The model under review builds one solid part; all positions refer to its coordinate system, in mm. A direction names the side the tool comes from. Round coordinates to 2 decimals unless told otherwise and drop trailing zeros. Write each loop counter-clockwise with the first axis right and the second up, starting at its lowest first coordinate (ties: lowest second). Pieces come first, ordered by that corner, then holes.
Item 1: Clearance check with flat-ended pins moving along their axes: pin 1 Ø2 at (x, z) = (3, -18) entering from +Y; pin 2 Ø10 at (x, z) = (1.5, -8) entering from -Y; pin 3 Ø1.6 at (x, z) = (0, -14.75) entering from +Y. State where each tip first meets the part, or that it passes through.
Item 2: To check wall thickness, follow L1, parallel to Y at x = 5.6, z = -5; L2, parallel to X at y = -5.6, z = -5; L3, parallel to X at y = 12.5, z = -3. State the ranges of each line that lie inside material, in increasing order.
Item 3: Draft analysis for pull direction Z (two halves, no side actions). For faces 1 (the face through (-0.492, -3.948, -15.521)), 2 (the face through (5, 0, -20)), 3 (the face through (3.948, 8.939, -5.422)), state which applies: +Z half, -Z half, draft (parallel to the pull), parting line (faces both ways), or undercut.
Item 4: Machinability: for faces 4 (the face through (0, 10, 0.5)), 5 (the face through (5, 2.75, -15)), 6 (the face through (4.4, -2.81, -10.22)), 7 (the face through (3.5, 0, -15)), which of the approach directions +Z, -Z, +X, -X, +Y, -Y give a long, thin tool a straight path to every point of the face, cutting with its end or side? Answer none if there is none.
Item 5: Add section A-A (y = 11.75). Give the boundary of the cut face in (x, z).
```python
from build123d import *

# Parameters (mm, degrees)
BOSS_EXTRUDE1_DEPTH           = 0.5
SKETCH6_R                     = 1.1
BOSS_EXTRUDE3_DEPTH           = 1.5
BOSS_EXTRUDE3_TAPER           = 10
BOSS_EXTRUDE3_OTHER_WAY_DEPTH = 1.5
BOSS_EXTRUDE3_OTHER_WAY_TAPER = 10
CHAMFER1_SIZE                 = 0.24656061
CHAMFER1_SIZE_2               = 0.2
CIRPATTERN2_COUNT             = 2
CIRPATTERN2_ANGLE             = 270
CIRPATTERN3_COUNT             = 2
CIRPATTERN3_ANGLE             = 90
CUT_EXTRUDE8_DEPTH            = 33.330326321
CUT_EXTRUDE10_DEPTH           = 30.5
CUT_EXTRUDE11_DEPTH           = 33.330326321
SKETCH8_R                     = 1.35
SKETCH8_R_2                   = 1.01183651
BOSS_EXTRUDE4_DEPTH           = 0.15
SKETCH12_R                    = 1.35
SKETCH12_R_2                  = 1.01183651
BOSS_EXTRUDE5_DEPTH           = 0.15
SKETCH13_R                    = 1.35
SKETCH13_R_2                  = 1.01183651
BOSS_EXTRUDE6_DEPTH           = 0.15
SKETCH2_R                     = 1.35
BOSS_EXTRUDE2_DEPTH           = 1
FILLET1_R                     = 1
CUT_EXTRUDE2_DEPTH            = 34.638240887
CUT_EXTRUDE4_DEPTH            = 32.129266776
CUT_EXTRUDE6_DEPTH            = 4


with BuildPart() as part:
    # Sketch1 → Boss-Extrude1 (new, symmetric)
    with BuildSketch(Plane.XY):
        Polygon((-5, 2.75), (-5, 5), (-2.75, 5), (-2.75, 15), (2.75, 15), (2.75, 5), (-5, -2.75), (-15, -2.75), (-15, 2.75), align=None)
    extrude(amount=BOSS_EXTRUDE1_DEPTH, both=True)

    # Sketch6 → Boss-Extrude3 (add)
    with BuildSketch(Plane(origin=(0, -0.5, 0), x_dir=(-1, 0, 0), z_dir=(0, 0, -1))):
        with Locations((0, 10.25)):
            Circle(SKETCH6_R)
        with Locations((9.75, 0.5)):
            Circle(SKETCH6_R)
    extrude(amount=BOSS_EXTRUDE3_DEPTH, taper=BOSS_EXTRUDE3_TAPER)

    # Sketch6 → Boss-Extrude3 other way (add)
    with BuildSketch(Plane(origin=(0, -0.5, 0), x_dir=(-1, 0, 0), z_dir=(0, 0, -1))):
        with Locations((0, 10.25)):
            Circle(SKETCH6_R)
        with Locations((9.75, 0.5)):
            Circle(SKETCH6_R)
    extrude(amount=-BOSS_EXTRUDE3_OTHER_WAY_DEPTH, taper=BOSS_EXTRUDE3_OTHER_WAY_TAPER)

    # Chamfer1
    # the kernel refuses this chamfer: 0.24656061, 0.2 mm, written as the material it takes off along each edge
    with BuildSketch(Plane(origin=(0, 9.75, 1.5), x_dir=(-1, 0, 0), z_dir=(0, -1, 0))) as chamfer1_piece_1:
        Polygon((0.835509529 + CHAMFER1_SIZE * 0.173648177924, CHAMFER1_SIZE * 0.984807754467), (0.835509529 - CHAMFER1_SIZE_2, 0), (0.835509529, 0), align=None)
    revolve(axis=Axis((0, 9.75, 1.5), (0, 0, -1)), mode=Mode.SUBTRACT)
    with BuildSketch(Plane(origin=(0, 9.75, -1.5), x_dir=(-1, 0, 0), z_dir=(0, 1, 0))) as chamfer1_piece_2:
        Polygon((0.835509529 + CHAMFER1_SIZE_2 * 0.173648177667, CHAMFER1_SIZE_2 * 0.984807753012), (0.835509529 - CHAMFER1_SIZE * 1.00000000148, 0), (0.835509529, 0), align=None)
    revolve(axis=Axis((0, 9.75, -1.5), (0, 0, 1)), mode=Mode.SUBTRACT)
    with BuildSketch(Plane(origin=(-9.75, 0, 1.5), x_dir=(-1, 0, 0), z_dir=(0, -1, 0))) as chamfer1_piece_3:
        Polygon((0.835509529 + CHAMFER1_SIZE * 0.173648177924, CHAMFER1_SIZE * 0.984807754467), (0.835509529 - CHAMFER1_SIZE_2, 0), (0.835509529, 0), align=None)
    revolve(axis=Axis((-9.75, 0, 1.5), (0, 0, -1)), mode=Mode.SUBTRACT)
    with BuildSketch(Plane(origin=(-9.75, 0, -1.5), x_dir=(-1, 0, 0), z_dir=(0, 1, 0))) as chamfer1_piece_4:
        Polygon((0.835509529 + CHAMFER1_SIZE_2 * 0.173648177667, CHAMFER1_SIZE_2 * 0.984807753012), (0.835509529 - CHAMFER1_SIZE * 1.00000000148, 0), (0.835509529, 0), align=None)
    revolve(axis=Axis((-9.75, 0, -1.5), (0, 0, 1)), mode=Mode.SUBTRACT)


with BuildPart() as cirpattern2_1:
    # CirPattern2: pattern copy
    add(part.part.rotate(Axis((0, -5, 0), (1, 0, 0)), 1 * CIRPATTERN2_ANGLE / (CIRPATTERN2_COUNT - 1)))

    # Sketch9 → Cut-Extrude8 (cut, through all)
    with BuildSketch(Plane.XZ.offset(5.5)):
        Polygon((-5, -10), (-2.75, -10), (-2.75, -20), (2.75, -20), (2.75, -10), (-5, -2.25), (-15, -2.25), (-15, -7.75), (-5, -7.75), align=None)
    extrude(amount=CUT_EXTRUDE8_DEPTH, mode=Mode.SUBTRACT)

    # Sketch12 → Boss-Extrude5 (add)
    # profile 1 of 2: a face of its own
    with BuildSketch(Plane.XZ.offset(5.5)):
        with Locations(Location((-9.75, -5, 0), (0, 0, 270))):
            Circle(SKETCH12_R)
        with Locations(Location((-9.75, -5, 0), (0, 0, 270))):
            Circle(SKETCH12_R_2, mode=Mode.SUBTRACT)
    # profile 2 of 2: a face of its own
    with BuildSketch(Plane.XZ.offset(5.5)):
        with Locations(Location((0, -14.75, 0), (0, 0, 270))):
            Circle(SKETCH12_R)
        with Locations(Location((0, -14.75, 0), (0, 0, 270))):
            Circle(SKETCH12_R_2, mode=Mode.SUBTRACT)
    extrude(amount=BOSS_EXTRUDE5_DEPTH)


with BuildPart() as cirpattern3_1:
    # CirPattern3: pattern copy
    add(part.part.rotate(Axis((5, 0, 0), (0, -1, 0)), 1 * CIRPATTERN3_ANGLE / (CIRPATTERN3_COUNT - 1)))

    # Sketch11 → Cut-Extrude11 (cut, through all)
    with BuildSketch(Plane(origin=(5.5, 0, 0), x_dir=(0, 0, -1), z_dir=(1, 0, 0))):
        Polygon((10, 5), (7.75, 5), (7.75, 15), (2.25, 15), (2.25, 5), (10, -2.75), (20, -2.75), (20, 2.75), (10, 2.75), align=None)
    extrude(amount=CUT_EXTRUDE11_DEPTH, mode=Mode.SUBTRACT)

    # Sketch13 → Boss-Extrude6 (add)
    # profile 1 of 2: a face of its own
    with BuildSketch(Plane(origin=(5.5, 0, 0), x_dir=(0, 0, -1), z_dir=(1, 0, 0))):
        with Locations((14.75, 0)):
            Circle(SKETCH13_R)
        with Locations((14.75, 0)):
            Circle(SKETCH13_R_2, mode=Mode.SUBTRACT)
    # profile 2 of 2: a face of its own
    with BuildSketch(Plane(origin=(5.5, 0, 0), x_dir=(0, 0, -1), z_dir=(1, 0, 0))):
        with Locations((5, 9.75)):
            Circle(SKETCH13_R)
        with Locations((5, 9.75)):
            Circle(SKETCH13_R_2, mode=Mode.SUBTRACT)
    extrude(amount=BOSS_EXTRUDE6_DEPTH)


with BuildPart() as part_1:
    add(part.part)

    # Sketch10 → Cut-Extrude10 (cut, through all)
    with BuildSketch(Plane.XY.offset(0.5)):
        Polygon((-2.75, 5), (-5, 5), (-5, 2.75), (-15, 2.75), (-15, -2.75), (-5, -2.75), (2.75, 5), (2.75, 15), (-2.75, 15), align=None)
    extrude(amount=CUT_EXTRUDE10_DEPTH, mode=Mode.SUBTRACT)

    # Sketch8 → Boss-Extrude4 (add)
    # profile 1 of 2: a face of its own
    with BuildSketch(Plane.XY.offset(0.5)):
        with Locations(Location((-9.75, 0, 0), (0, 0, 180))):
            Circle(SKETCH8_R)
        with Locations((-9.75, 0)):
            Circle(SKETCH8_R_2, mode=Mode.SUBTRACT)
    # profile 2 of 2: a face of its own
    with BuildSketch(Plane.XY.offset(0.5)):
        with Locations(Location((0, 9.75, 0), (0, 0, 180))):
            Circle(SKETCH8_R)
        with Locations((0, 9.75)):
            Circle(SKETCH8_R_2, mode=Mode.SUBTRACT)
    extrude(amount=BOSS_EXTRUDE4_DEPTH)

    add(cirpattern2_1.part)  # Boss-Extrude2 merges CirPattern2_1

    add(cirpattern3_1.part)  # Boss-Extrude2 merges CirPattern3_1
    # Sketch2 → Boss-Extrude2 (add)
    with BuildSketch(Plane(origin=(-0.583333333, 0.583333333, -0.583333333), x_dir=(0.8164965809277334, 0.4082482904638652, -0.40824829046384614), z_dir=(-0.5773502691896154, 0.5773502691896445, -0.5773502691896175))):
        Polygon((7.450531301, 9.01561146), (7.450531301, -1.944543648), (4.082482905, -3.889087297), (-5.409289849, 1.590990258), (-5.409289849, 5.480077554), (4.082482905, 10.960155108), align=None)
        with Locations(Location((2.041241452, 3.535533906, 0), (0, 0, 270))):
            Circle(SKETCH2_R, mode=Mode.SUBTRACT)
    extrude(amount=BOSS_EXTRUDE2_DEPTH)

    # Fillet1
    fillet1_edges = [part_1.edges().sort_by_distance(p)[0] for p in [
        (-1.125, 1.125, 0.5),
        (-1.125, -5.5, -6.125),
        (5.5, 1.125, -6.125),
    ]]
    fillet(fillet1_edges, radius=FILLET1_R)

    # Sketch3 → Cut-Extrude2 (cut, through all)
    with BuildSketch(Plane(origin=(4.125, -4.125, 0), x_dir=(0.7071067811865475, 0.7071067811865477, -2.769222492809729e-15), z_dir=(-0.7071067811865477, 0.7071067811865475, -2.769222492809729e-15))):
        with BuildLine():
            Line((1.125, 10), (1.125, 11.125))
            Line((1.125, 11.125), (-1.125, 11.125))
            Line((-1.125, 11.125), (-1.125, 10))
            ThreePointArc((-1.125, 10), (0, 8.875), (1.125, 10))
        make_face()
    extrude(amount=CUT_EXTRUDE2_DEPTH, mode=Mode.SUBTRACT)

    # Sketch4 → Cut-Extrude4 (cut, through all)
    with BuildSketch(Plane(origin=(1.625, 0, 1.625), x_dir=(-0.7071067811865487, 2.4677036874675166e-14, 0.7071067811865465), z_dir=(-0.7071067811865465, -2.4677036874675254e-14, -0.7071067811865487))):
        with BuildLine():
            Line((-2.410533906, 5), (-2.410533906, 6.125))
            Line((-2.410533906, 6.125), (-4.660533906, 6.125))
            Line((-4.660533906, 6.125), (-4.660533906, 5))
            ThreePointArc((-4.660533906, 5), (-3.535533906, 3.875), (-2.410533906, 5))
        make_face()
    extrude(amount=CUT_EXTRUDE4_DEPTH, mode=Mode.SUBTRACT)

    # Sketch5 → Cut-Extrude6 (cut)
    with BuildSketch(Plane(origin=(0, -1.625, 1.625), x_dir=(-1, 0, 0), z_dir=(-5.877305542968418e-15, 0.7071067811865465, -0.7071067811865486))):
        with BuildLine():
            Line((5, -4.660533906), (6.125, -4.660533906))
            Line((6.125, -4.660533906), (6.125, -2.410533906))
            Line((6.125, -2.410533906), (5, -2.410533906))
            ThreePointArc((5, -2.410533906), (3.875, -3.535533906), (5, -4.660533906))
        make_face()
    extrude(amount=CUT_EXTRUDE6_DEPTH, mode=Mode.SUBTRACT)


solid = part_1.part
```
Numbers:
1. pin 1: stops at y = -4.5
1. pin 2: stops at y = -5.5
1. pin 3: stops at y = -3.5
2. L1: y = 8.4 to 8.74, 10.76 to 11.1
2. L2: x = -11.1 to -10.76, -8.74 to -8.4
2. L3: x = 4.5 to 5.5
3. face 1: undercut
3. face 2: -Z half
3. face 3: parting line
4. face 4: +Z
4. face 5: -Z, +X, -X, +Y
4. face 6: -Z, -X, -Y
4. face 7: -Z, -X, +Y, -Y
5. outline: (-2.75, -0.5) - (2.75, -0.5) - (2.75, 0.5) - (-2.75, 0.5) - close; (4.5, -7.75) - (5.5, -7.75) - (5.5, -2.25) - (4.5, -2.25) - close
